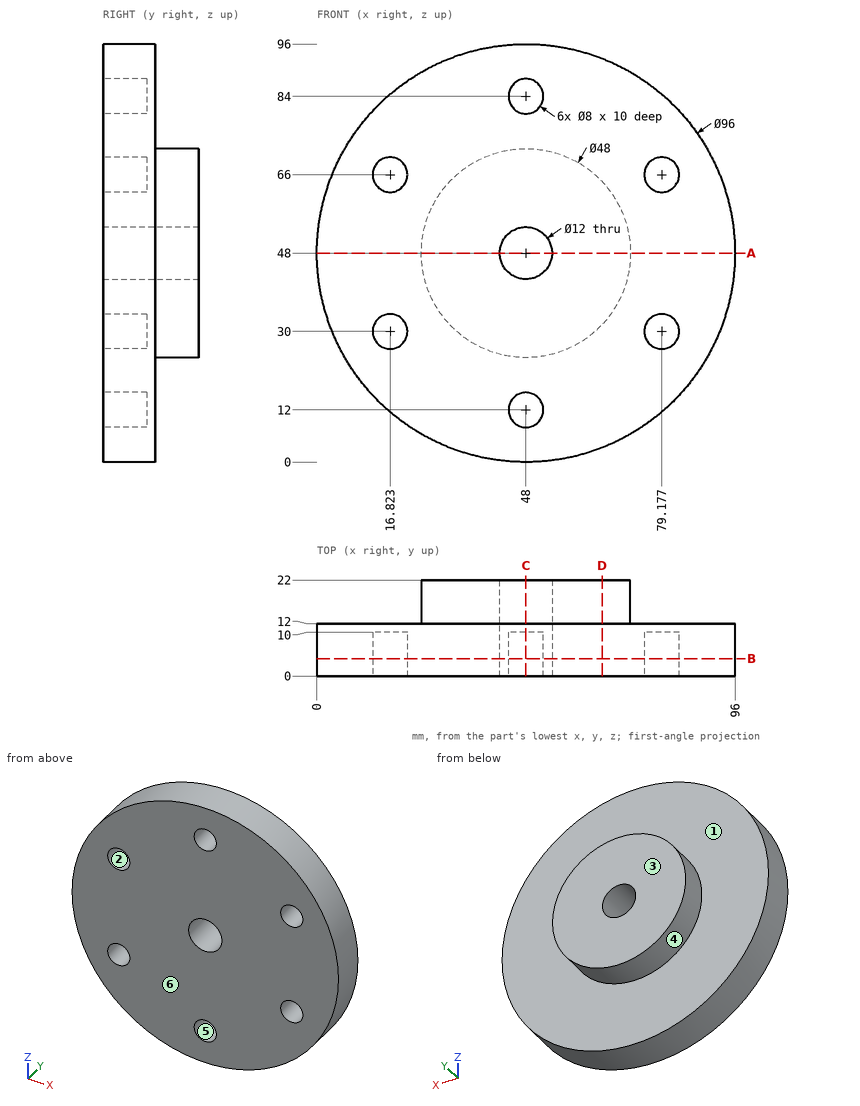
For this review, use the dimensioned drawing (mm, ordinates from the lowest corner) and the shaded views. A direction names the side the tool comes from. Give positions to 0.01 mm unless a question says otherwise; leave off trailing zeros. Write each loop counter-clockwise with the first axis right and the second up, starting at its lowest first coordinate (ties: lowest second). Pieces come first, ordered by that corner, then holes.
(1) For P1, Ø9, axis at x = 47, z = 82.5, coming from the -Y side; P2, Ø4, axis at x = 16.5, z = 28.5, coming from the -Y side; P3, Ø12, axis at x = 37, y = 2, coming from the -Z side; P4, Ø3, axis at x = 69.5, y = 17.5, coming from the +Z side, all flat-tipped, find the tip position at first contact; note any pin that passes through.
(2) Consider section D-D, the plane x = 65.5. Give the boundary of the cut face in (y, z), and give its area (3 significant figures).
(3) To check wall thickness, follow L1, parallel to Z at x = 16, y = 1.5; L2, parallel to Z at x = 48, y = 7.25; L3, parallel to X at y = 11.25, z = 48. State the ranges of each line that lie inside material, in increasing order.
(4) Consider section C-C, the plane x = 48. Give the boundary of the cut face in (y, z).
(5) Tool access review of the marked faces 1, 2 and 3: name each direction out of +Z, -Z, +X, -X, +Y, -Y from which nothing blocks a thin tool from reaching the whole face with its end or side.
(6) Consider section B-B, the plane y = 4. Give the boundary of the cut face in (x, z), and give its area (3 significant figures).
(7) Consider section A-A, the plane z = 48. Give the boundary of the cut face in (x, y), and give its area (3 significant figures).
(8) The part is to be moulded in two halves that separate along Z. For the marked faces 4, 5 and 6, say which applies: released by +Z, released by -Z, zero draft, split by the parting line, or undercut.
Returned:
1. P1: stops at y = 0
1. P2: stops at y = 10
1. P3: stops at z = 0.26
1. P4: stops at z = 61.27
2. outline: (0, 3.3) - (12, 3.3) - (12, 31.58) - (22, 31.58) - (22, 64.42) - (12, 64.42) - (12, 92.7) - (0, 92.7) - close
2. area: 1,400 mm2
3. L1: z = 12.22 to 26.09, 33.91 to 62.09, 69.91 to 83.78
3. L2: z = 0 to 8, 16 to 42, 54 to 80, 88 to 96
3. L3: x = 0 to 42, 54 to 96
4. outline: (0, 0) - (12, 0) - (12, 24) - (22, 24) - (22, 42) - (0, 42) - (0, 16) - (10, 16) - (10, 8) - (0, 8) - close; (0, 54) - (22, 54) - (22, 72) - (12, 72) - (12, 96) - (0, 96) - (0, 88) - (10, 88) - (10, 80) - (0, 80) - close
5. face 1: +Y
5. face 2: -Y
5. face 3: +Z, -Z, +X, -X, +Y
6. outline: circle Ø96 at (48, 48); hole circle Ø8 at (16.82, 30); hole circle Ø8 at (16.82, 66); hole circle Ø12 at (48, 48); hole circle Ø8 at (48, 12); hole circle Ø8 at (48, 84); hole circle Ø8 at (79.18, 30); hole circle Ø8 at (79.18, 66)
6. area: 6,820 mm2
7. outline: (0, 0) - (42, 0) - (42, 22) - (24, 22) - (24, 12) - (0, 12) - close; (54, 0) - (96, 0) - (96, 12) - (72, 12) - (72, 22) - (54, 22) - close
7. area: 1,370 mm2
8. face 4: split by the parting line
8. face 5: undercut
8. face 6: zero draft
